CAD build for the part. Positions are in the model's coordinates, mm. A direction names the side the tool comes from. Coordinates: 2 decimals unless noted, no trailing zeros. Order: outer loops, then holes, each group sorted by start corner. A loop starts at its lowest first (then second) coordinate and runs counter-clockwise, first axis right, second up. Notation, with made-up numbers: (59.5, 27) - (74.5, 27) arc R23 ccw to (74.5, 43) - close; hole circle Ø6 at (57, 69). An arc over 180 degrees is marked (long way). Write each question's results on one line, items separated by ' | '. Start each with the question number.
Q1. Wall check: probe 1 along Y at (x, z) = (24.25, 0.8); probe 2 along X at (y, z) = (-38, 18.25); probe 3 along Z at (x, y) = (5, -2). Give the ranges that are in metal, low to high.
Q2. Which spindle directions (+Z, -Z, +X, -X, +Y, -Y) get a long thin tool onto all of the face, cutting with end or side? Do faces 4 (the flat face through (0, -10, 3)), 5 (the cylindrical face through (-21.235, -36.064, 2.149)). Say none if no direction does.
Q3. Band-saw the part on D-D, the plane y = -10.5. Write the cut outline in (x, z).
Q4. Pull direction Z, two halves, no side cores. Call faces 1 (the flat face through (-0.381, -29.763, 12.947)), 2 (the cylindrical face through (24, -36, 3)), 3 (the flat face through (0, 0, 1)): released by +Z, released by -Z, zero draft, split by the parting line, or undercut.
Q5. Pin check, flat tips, straight feed: P1, Ø6, axis at x = 1.5, y = -8, coming from the +Z side; P2, Ø1.5, axis at x = -9, z = 7.5, coming from the -Y side; P3, Ø10, axis at x = 9.5, y = -16.5, coming from the +Z side. Stop position of each tip, or through.
Q6. Band-saw the part on C-C, the plane z = 19. Count the separate pieces of the cut face and the enclosed holes in it, then the cut area to 3 significant figures.
Q7. Band-saw the part on A-A, the plane y = -15. Write the cut outline in (x, z), then the cut area to 3 significant figures.
Q8. Band-saw the part on B-B, the plane x = 8.5. Write the cut outline in (y, z).
```python
from build123d import *

# Parameters (mm, degrees)
SKETCH_1_W          = 54.5
SKETCH_1_H          = 40
SKETCH_1_R          = 2.1
EXTRUDE_1_DEPTH     = 3
EXTRUDE_2_DEPTH     = 54.5
SKETCH_3_R          = 1.5
SKETCH_3_R_2        = 1.6
CUT_EXTRUDE_1_DEPTH = 8
CUT_EXTRUDE_START   = -10
SKETCH_4_R          = 4
CUT_EXTRUDE_2_DEPTH = 7


with BuildPart() as part:
    # 草图1 → 凸台-拉伸1 (new body)
    with BuildSketch(Plane.XY):
        with Locations((0, -20)):
            Rectangle(SKETCH_1_W, SKETCH_1_H)
        with Locations((-24.25, -5)):
            Circle(SKETCH_1_R, mode=Mode.SUBTRACT)
        with Locations(Location((24.25, -5, 0), (0, 0, 180))):
            Circle(SKETCH_1_R, mode=Mode.SUBTRACT)
        with Locations((24.25, -15)):
            Circle(SKETCH_1_R, mode=Mode.SUBTRACT)
        with Locations(Location((-24.25, -15, 0), (0, 0, 180))):
            Circle(SKETCH_1_R, mode=Mode.SUBTRACT)
    extrude(amount=EXTRUDE_1_DEPTH)

    # 草图2 → 凸台-拉伸2 (add)
    with BuildSketch(Plane.ZY.offset(27.25)):
        Polygon((3, -20), (23.176339002, -39.802940776), (3, -40), align=None)
    extrude(amount=-EXTRUDE_2_DEPTH)

    # 草图3 → 切除-拉伸1 (cut)
    with BuildSketch(Plane(origin=(0, -40.025482459, 0.390922779), x_dir=(1, 0, 0), z_dir=(0, -0.9999523077580083, 0.009766381593687423))):
        with Locations(Location((-22.5, 2.602610467, 0), (0, 0, 270))):
            Circle(SKETCH_3_R)
        with Locations(Location((-22.5, 17.602610467, 0), (0, 0, 270))):
            Circle(SKETCH_3_R_2)
        with Locations(Location((22.5, 17.602610467, 0), (0, 0, 270))):
            Circle(SKETCH_3_R_2)
        with Locations(Location((22.5, 2.602610467, 0), (0, 0, 270))):
            Circle(SKETCH_3_R)
    extrude(amount=-CUT_EXTRUDE_1_DEPTH, mode=Mode.SUBTRACT)

    # 草图4 → 切除-拉伸2 (cut)
    with BuildSketch(Plane(origin=(0, -40.025482459, 0.390922779), x_dir=(1, 0, 0), z_dir=(0, -0.9999523077580083, 0.009766381593687423)).offset(CUT_EXTRUDE_START)):
        with Locations((-22.5, 17.602610467)):
            Circle(SKETCH_4_R)
        with Locations((22.5, 17.602610467)):
            Circle(SKETCH_4_R)
    extrude(amount=CUT_EXTRUDE_2_DEPTH, mode=Mode.SUBTRACT)


solid = part.part
```
Results below:
1) probe 1: y = -40 to -17.1, -12.9 to -7.1, -2.9 to 0 | probe 2: x = -27.25 to -24.08, -20.92 to 20.92, 24.08 to 27.25 | probe 3: z = 0 to 3
2) face 4: +Z, +X, -X, +Y | face 5: none
3) outline: (-27.25, 0) - (27.25, 0) - (27.25, 3) - (-27.25, 3) - close
4) face 1: released by +Z | face 2: undercut | face 3: zero draft
5) P1: stops at z = 3 | P2: stops at y = -39.96 | P3: stops at z = 4.53
6) separate pieces: 3 | enclosed holes: 0 | area: 193 mm²
7) outline: (-27.25, 0) - (-26.35, 0) - (-26.35, 3) - (-27.25, 3) - close; (-22.15, 0) - (22.15, 0) - (22.15, 3) - (-22.15, 3) - close; (26.35, 0) - (27.25, 0) - (27.25, 3) - (26.35, 3) - close | area: 138 mm²
8) outline: (-40, 0) - (0, 0) - (0, 3) - (-20, 3) - (-39.8, 23.18) - (-40, 3) - close
